Design review of the part built by this model. Coordinates are the model's own, in mm. Face numbers are marked on the shaded views. A direction names the side the tool comes from. Round coordinates to 2 decimals unless told otherwise and drop trailing zeros. Write each loop counter-clockwise with the first axis right and the second up, starting at its lowest first coordinate (ties: lowest second). Pieces come first, ordered by that corner, then holes. Notation, with made-up numbers: (-25, 26) -> (9, 26) arc R31 cw to (9, 54) -> close; hole circle Ø8 at (16.5, 11). An arc over 180 degrees is marked (long way). One line per question, with ' | ' between items. Start each with the question number.
1) For the marked faces 1, 2 and 3, list the 3-axis set-ups (+Z, -Z, +X, -X, +Y, -Y) from which the entire face can be reached by the end or side of a thin tool; tool diameter is ignored.
2) Mouldability with a two-part tool opening along Y and no side actions: class the marked faces 4, 5 and 6 as +Y half, -Y half, draft (parallel to the pull), parting line (faces both ways), or undercut.
3) Consider section C-C (y = 36). Give the boundary of the cut face in (x, z), then the cut area to 3 significant figures.
4) Consider section A-A (y = 20). Give the boundary of the cut face in (x, z).
5) For probe 1 along Y at (x, z) = (68.5, 27); probe 2 along Y at (x, z) = (51, 24.5); probe 3 along Y at (x, z) = (54, 21.25), list the stretches that pass through material, from the lowest coordinate up.
6) Insertion check: pin 1 Ø8 at (x, y) = (4, 36) entering from +Z; pin 2 Ø3 at (x, y) = (46, 4) entering from +Z; pin 3 Ø4 at (x, y) = (4, 4) entering from +Z. Each pin has a flat end and moves straight along its axis. Give the tip position at first contact, or say it passes through.
7) Consider section B-B (x = 24.5). Give the boundary of the cut face in (y, z), then the cut area to 3 significant figures.
8) Consider section D-D (x = 46). Count the separate pieces of the cut face and the enclosed holes in it, then the cut area to 3 significant figures.
```python
from build123d import *

# Parameters (mm, degrees)
SKETCH292_W     = 100
SKETCH292_H     = 50
SKETCH292_R     = 14
SKETCH292_R_2   = 1.75
SKETCH292_R_3   = 1.65
PAD139_DEPTH    = 8
SKETCH293_W     = 100
SKETCH293_H     = 12.25
POCKET126_DEPTH = 4
POCKET127_DEPTH = 8.001
SKETCH295_R     = 3.5
POCKET128_DEPTH = 2


with BuildPart() as part:
    # Sketch292 → Pad139 (new body)
    with BuildSketch(Plane.XY):
        with Locations((50, 25)):
            Rectangle(SKETCH292_W, SKETCH292_H)
        with Locations((50, 25)):
            Circle(SKETCH292_R, mode=Mode.SUBTRACT)
        with Locations((29, 41)):
            Circle(SKETCH292_R_2, mode=Mode.SUBTRACT)
        with Locations((71, 41)):
            Circle(SKETCH292_R_2, mode=Mode.SUBTRACT)
        with Locations((71, 9)):
            Circle(SKETCH292_R_2, mode=Mode.SUBTRACT)
        with Locations((29, 9)):
            Circle(SKETCH292_R_2, mode=Mode.SUBTRACT)
        with Locations((96.5, 33.25)):
            Circle(SKETCH292_R_3, mode=Mode.SUBTRACT)
        with Locations((3.5, 33.25)):
            Circle(SKETCH292_R_3, mode=Mode.SUBTRACT)
        with Locations((3.5, 16.75)):
            Circle(SKETCH292_R_3, mode=Mode.SUBTRACT)
        with Locations((96.5, 16.75)):
            Circle(SKETCH292_R_3, mode=Mode.SUBTRACT)
    extrude(amount=PAD139_DEPTH)

    # Sketch293 (on Face15 of Pad139) → Pocket126 (cut)
    with BuildSketch(Plane.XY.offset(8)):
        with Locations((50, 41.875)):
            Rectangle(SKETCH293_W, SKETCH293_H)
        with Locations((50, 8.125)):
            Rectangle(SKETCH293_W, SKETCH293_H)
    extrude(amount=-POCKET126_DEPTH, mode=Mode.SUBTRACT)

    # Sketch294 (on Face9 of Pocket126) → Pocket127 (cut, through all)
    with BuildSketch(Plane.XY.offset(8)):
        with BuildLine():
            ThreePointArc((11, 33), (3, 25), (11, 17))
            Line((11, 17), (26, 17))
            ThreePointArc((26, 17), (34, 25), (26, 33))
            Line((26, 33), (11, 33))
        make_face()
        with BuildLine():
            ThreePointArc((74, 33), (66, 25), (74, 17))
            Line((74, 17), (89, 17))
            ThreePointArc((89, 17), (97, 25), (89, 33))
            Line((89, 33), (74, 33))
        make_face()
    extrude(amount=-POCKET127_DEPTH, mode=Mode.SUBTRACT)

    # Sketch295 (on Face11 of Pocket127) → Pocket128 (cut)
    with BuildSketch(Plane.XY.offset(4)):
        with Locations((29, 41)):
            Circle(SKETCH295_R)
        with Locations((71, 41)):
            Circle(SKETCH295_R)
        with Locations((29, 9)):
            Circle(SKETCH295_R)
        with Locations((71, 9)):
            Circle(SKETCH295_R)
    extrude(amount=-POCKET128_DEPTH, mode=Mode.SUBTRACT)


with BuildPart() as part_1:
    # Body103 placement: moved
    add(part.part.moved(Location((-25, -5, 20))))


solid = part_1.part
```
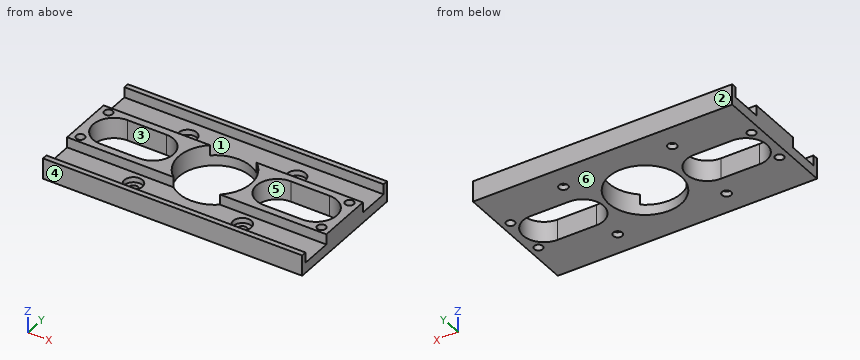
From the geometry:
1) face 1: +Z, +X, -X | face 2: +Z, -Z, +X, -X, +Y | face 3: +Z, -Z
2) face 4: -Y half | face 5: undercut | face 6: draft
3) outline: (-25, 20) -> (2.25, 20) -> (2.25, 22) -> (0.5, 22) -> (0.5, 24) -> (-25, 24) -> close; (5.75, 20) -> (44.25, 20) -> (44.25, 22) -> (42.5, 22) -> (42.5, 24) -> (7.5, 24) -> (7.5, 22) -> (5.75, 22) -> close; (47.75, 20) -> (75, 20) -> (75, 24) -> (49.5, 24) -> (49.5, 22) -> (47.75, 22) -> close | area: 358 mm2
4) outline: (-25, 20) -> (-22, 20) -> (-22, 28) -> (-25, 28) -> close; (9, 20) -> (11, 20) -> (11, 28) -> (9, 28) -> close; (39, 20) -> (41, 20) -> (41, 28) -> (39, 28) -> close; (72, 20) -> (75, 20) -> (75, 28) -> (72, 28) -> close
5) probe 1: y = -5 to -3, 9.25 to 13.39, 26.61 to 30.75, 43 to 45 | probe 2: y = -5 to -3, 9.25 to 12, 28 to 30.75, 43 to 45 | probe 3: y = -5 to 12, 28 to 45
6) pin 1: stops at z = 24 | pin 2: passes through | pin 3: stops at z = 22
7) outline: (-5, 20) -> (6.01, 20) -> (6.01, 24) -> (-3, 24) -> (-3, 28) -> (-5, 28) -> close; (33.99, 20) -> (45, 20) -> (45, 28) -> (43, 28) -> (43, 24) -> (33.99, 24) -> close | area: 104 mm2
8) separate pieces: 4 | enclosed holes: 0 | area: 141 mm2
